Build history of the part. All positions in model axes, mm. Face numbers are marked on the shaded views. Give positions to 0.01 mm unless a question says otherwise; leave off trailing zeros. Loops run counter-clockwise (first coordinate to the right, second up) from the corner with the lowest first, then second, coordinate; pieces in that order, holes last. Notation, with made-up numbers: M 59,-3.5 L 73,-3.5 A21 ccw 73,4.5 Z; hole C 47.25,13.5 d1. An arc over 180 degrees is marked long. Answer as a JSON object with one key per item and string values. Group by question number.
1. Mould opens along Z. For the marked faces 1 and 2 say: released by +Z, released by -Z, zero draft, split by the parting line, or undercut.
2. Drill centre lines: line 1 along Y through (x, z) = (18.4, 0); line 2 along Z through (x, y) = (31, 0.25); line 3 along Y through (x, z) = (6.5, 0). Where is each one in solid material? Low to high. Write a range as [from, to].
3. Drop flat-ended pins along their axis: pin 1 Ø6 at (y, z) = (-1, -4) entering from -X; pin 2 Ø1.5 at (x, y) = (24.5, -4) entering from -Z; pin 3 Ø4 at (x, y) = (23, -4) entering from +Z. Give the stop position or say it passes through.
4. Slice it at D-D (x = 13). List the corners of the cut face in (y, z), then the cut area to 3 significant figures.
5. Slice it at C-C (x = 6.5). List the corners of the cut face in (y, z), then the cut area to 3 significant figures.
from build123d import *

# Parameters (mm, degrees)
SKETCH1_R           = 5.55625
SKETCH1_R_2         = 4.5593
BOSS_EXTRUDE1_DEPTH = 35.56


with BuildPart() as part:
    # Sketch1 → Boss-Extrude1 (new body)
    with BuildSketch(Plane(origin=(0, 0, 0), x_dir=(0, 0, -1), z_dir=(1, 0, 0))):
        Circle(SKETCH1_R)
        Circle(SKETCH1_R_2, mode=Mode.SUBTRACT)
    extrude(amount=BOSS_EXTRUDE1_DEPTH)

    # Sketch2 → Cut-Revolve1 (revolve, cut)
    with BuildSketch(Plane.XY, mode=Mode.PRIVATE) as cut_revolve1_sk:
        Polygon((17.570232791, -4.445), (20.033534416, -4.445), (19.583193844, -4.976009125), (18.020573363, -4.976009125), align=None)
        Polygon((28.774465682, -4.445), (31.559150182, -4.445), (31.020477762, -5.004932574), (29.313138102, -5.004932574), align=None)
        Polygon((4.182688786, -4.445), (7.557077958, -4.445), (7.106737387, -5.18020875), (4.633029357, -5.18020875), align=None)
    revolve(cut_revolve1_sk.sketch.rotate(Axis((0, 0, 0), (1, 0, 0)), 270), axis=Axis((0, 0, 0), (1, 0, 0)), mode=Mode.SUBTRACT)


solid = part.part
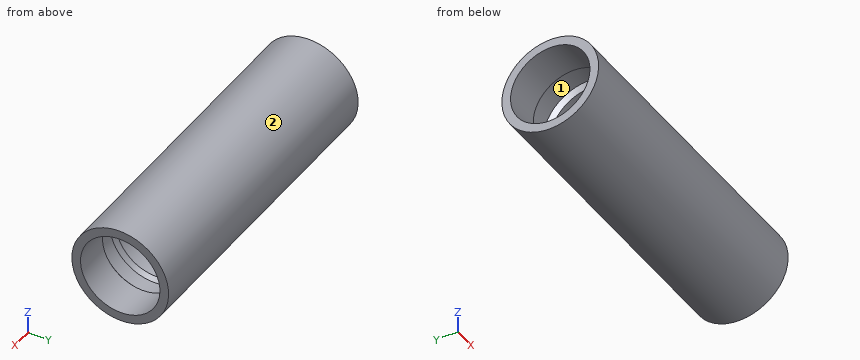
Established:
{
 "1": {"face 1": "undercut", "face 2": "split by the parting line"},
 "2": {"line 1": "y = [-5.56, -4.98], [4.98, 5.56]", "line 2": "z = [-5.55, -5], [5, 5.55]", "line 3": "y = [-5.56, -5.18], [5.18, 5.56]"},
 "3": {"pin 1": "stops at x = 0", "pin 2": "stops at z = -4.51", "pin 3": "stops at z = 5.18"},
 "4": {"outline": "C 0,0 d11.11; hole C 0,0 d9.12", "area": "31.7 mm^2"},
 "5": {"outline": "C 0,0 d11.11; hole C 0,0 d10.36", "area": "12.7 mm^2"}
}
